Verification items for the finished model (mm, model axes). A direction names the side the tool comes from. Coordinates: 2 decimals unless noted, no trailing zeros. Order: outer loops, then holes, each group sorted by start corner. A loop starts at its lowest first (then second) coordinate and runs counter-clockwise, first axis right, second up. Notation, with made-up numbers: (39, 0.5) -> (76, 0.5) arc R33 ccw to (76, 30.5) -> close; hole circle Ø2 at (69.5, 23). An arc over 180 degrees is marked (long way). Answer as CSV lines item,"result".
```python
from build123d import *

# Parameters (mm, degrees)
EXTRUDE_1_DEPTH          = 82
FILLET_1_R               = 3
EXTRUDE_2_DEPTH          = 10
SKETCH_3_R               = 8
SKETCH_3_R_2             = 5
CUT_EXTRUDE_1_DEPTH      = 42
CUT_EXTRUDE_1_DEPTH_BACK = 42
FILLET_2_R               = 15
SKETCH_4_R               = 5.5
CUT_EXTRUDE_2_DEPTH      = 97
CUT_EXTRUDE_2_DEPTH_BACK = 1
FILLET_3_R               = 3
FILLET_4_R               = 3


with BuildPart() as part:
    # 스케치1 → 보스-돌출1 (new body)
    with BuildSketch(Plane.XY):
        Polygon((0, 0), (-150, 0), (-150, 10), (-10, 10), (-10, 45), (0, 45), align=None)
    extrude(amount=-EXTRUDE_1_DEPTH)

    # 필렛1
    fillet_1_edges = [part.edges().sort_by_distance(p)[0] for p in [
        (-10, 45, -41),
    ]]
    fillet(fillet_1_edges, radius=FILLET_1_R)

    # 스케치2 → 보스-돌출2 (add)
    with BuildSketch(Plane(origin=(0, 0, -61), x_dir=(-1, 0, 0), z_dir=(0, 0, -1))):
        with BuildLine():
            Line((150, 0), (150, 25))
            Line((150, 25), (42, 40))
            Line((42, 40), (42, 75))
            ThreePointArc((42, 75), (21, 96), (0, 75))
            Line((0, 75), (0, 0))
            Line((0, 0), (150, 0))
        make_face()
    extrude_2 = extrude(amount=-EXTRUDE_2_DEPTH)

    # 대칭 복사1: 보스-돌출2 across plane
    add(extrude_2.mirror(Plane.XY.offset(-41)))

    # 스케치3 → 컷-돌출1 (cut, two sides)
    with BuildSketch(Plane.XY.offset(-41)) as cut_extrude_1_sk:
        with Locations((-21, 75)):
            Circle(SKETCH_3_R)
        with Locations((-135, 17.5)):
            Circle(SKETCH_3_R_2)
    extrude(amount=CUT_EXTRUDE_1_DEPTH, mode=Mode.SUBTRACT)
    extrude(cut_extrude_1_sk.sketch, amount=-CUT_EXTRUDE_1_DEPTH_BACK, mode=Mode.SUBTRACT)

    # 필렛2
    fillet_2_edges = [part.edges().sort_by_distance(p)[0] for p in [
        (-150, 25, -56),
        (-150, 25, -26),
    ]]
    fillet(fillet_2_edges, radius=FILLET_2_R)

    # 스케치4 → 컷-돌출2 (cut, two sides)
    with BuildSketch(Plane(origin=(0, 0, 0), x_dir=(1, 0, 0), z_dir=(0, 1, 0))) as cut_extrude_2_sk:
        with Locations((-30, 71.5)):
            Circle(SKETCH_4_R)
        with Locations((-90, 71.5)):
            Circle(SKETCH_4_R)
        with Locations((-30, 10.5)):
            Circle(SKETCH_4_R)
        with Locations((-90, 10.5)):
            Circle(SKETCH_4_R)
    extrude(amount=CUT_EXTRUDE_2_DEPTH, mode=Mode.SUBTRACT)
    extrude(cut_extrude_2_sk.sketch, amount=-CUT_EXTRUDE_2_DEPTH_BACK, mode=Mode.SUBTRACT)

    # 필렛3
    fillet_3_edges = [part.edges().sort_by_distance(p)[0] for p in [
        (-10, 10, -71.5),
        (-10, 10, -41),
        (-10, 10, -10.5),
    ]]
    fillet(fillet_3_edges, radius=FILLET_3_R)

    # 필렛4
    fillet_4_edges = [part.edges().sort_by_distance(p)[0] for p in [
        (-42, 40, -56),
        (-42, 40, -26),
    ]]
    fillet(fillet_4_edges, radius=FILLET_4_R)


solid = part.part
```
Item 1: Release check for a two-part mould opening along X. For faces 5 (the flat face through (-57, 34, -51)), 6 (the flat face through (-91.47, 33.13, -25.93)), 7 (the cylindrical face through (-22.041, 82.932, -26.07)) record: +X half, -X half, draft (parallel to the pull), parting line (faces both ways), or undercut.
Answer list:
face 5,"draft"
face 6,"-X half"
face 7,"undercut"
Item 2: Tool access check on faces 1 (the cylindrical face through (-10.9, 10.86, -41.14)), 2 (the flat face through (-42, 59, -56)), 3 (the flat face through (-82, 10, -71)), 4 (the flat face through (-4, 45, -10)). Record the directions out of +Z, -Z, +X, -X, +Y, -Y that give a thin tool (end or side, any length) a straight path to the whole face; none if there is none.
Answer list:
face 1,"-X, +Y"
face 2,"+Z, -Z, -X, +Y"
face 3,"-Z, -X, +Y"
face 4,"+Z, +X, -X, +Y"
Item 3: Thickness scan on line 1 (X direction, y = 3.25, z = -10.5); line 2 (Y direction, x = -21, z = -25.25); line 3 (Z direction, x = -90.5, y = 5). Record the ranges inside material, lowest first.
Answer list:
line 1,"-150 to -95.5, -84.5 to -35.5, -24.5 to 0"
line 2,"0 to 67, 83 to 96"
line 3,"-82 to -76.98, -66.02 to -15.98, -5.02 to 0"
Item 4: Section check A-A, the plane z = -71.5. Record the boundary of the cut face in (x, y), plus the area to 3 significant figures.
Answer list:
outline,"(-150, 0) -> (-95.5, 0) -> (-95.5, 10) -> (-150, 10) -> close; (-84.5, 0) -> (-35.5, 0) -> (-35.5, 10) -> (-84.5, 10) -> close; (-24.5, 0) -> (0, 0) -> (0, 45) -> (-7, 45) arc R3 ccw to (-10, 42) -> (-10, 13) arc R3 cw to (-13, 10) -> (-24.5, 10) -> close"
area,"1,630 mm2"
Item 5: Section check D-D, the plane y = 71. Record the boundary of the cut face in (x, z), plus the area to 3 significant figures.
Answer list:
outline,"(-42, -61) -> (-27.93, -61) -> (-27.93, -51) -> (-42, -51) -> close; (-42, -31) -> (-27.93, -31) -> (-27.93, -21) -> (-42, -21) -> close; (-14.07, -61) -> (0, -61) -> (0, -51) -> (-14.07, -51) -> close; (-14.07, -31) -> (0, -31) -> (0, -21) -> (-14.07, -21) -> close"
area,"563 mm2"
Item 6: Section check B-B, the plane x = -21. Record the boundary of the cut face in (y, z).
Answer list:
outline,"(0, -82) -> (10, -82) -> (10, -61) -> (67, -61) -> (67, -51) -> (10, -51) -> (10, -31) -> (67, -31) -> (67, -21) -> (10, -21) -> (10, 0) -> (0, 0) -> close; (83, -61) -> (96, -61) -> (96, -51) -> (83, -51) -> close; (83, -31) -> (96, -31) -> (96, -21) -> (83, -21) -> close"
Item 7: Section check C-C, the plane z = -58. Record the boundary of the cut face in (x, y), plus the area to 3 significant figures.
Answer list:
outline,"(-150, 0) -> (0, 0) -> (0, 75) arc R21 ccw to (-42, 75) -> (-42, 42.61) arc R3 cw to (-44.59, 39.64) -> (-137.06, 26.8) arc R15 ccw to (-150, 11.94) -> close; hole circle Ø10 at (-135, 17.5); hole circle Ø16 at (-21, 75)"
area,"7,040 mm2"
Item 8: Depth check by flat-ended pin: pin 1 Ø6 at (y, z) = (55.5, -25) entering from -X; pin 2 Ø17.5 at (x, z) = (-30, -10.5) entering from +Y; pin 3 Ø10 at (x, z) = (-106, -57.5) entering from +Y; pin 4 Ø4 at (x, z) = (-41, -13) entering from -Y. Enter the tip coordinate at first touch or a pass-through.
Answer list:
pin 1,"x = -42"
pin 2,"y = 10"
pin 3,"y = 31.81"
pin 4,"y = 0"
